Check sheet for the modelled part. Datum: model origin and axes. Units: mm. Face numbers are marked on the shaded views. A direction names the side the tool comes from. Give positions to 0.01 mm unless a question says otherwise; leave off trailing zeros. Loops run counter-clockwise (first coordinate to the right, second up) from the corner with the lowest first, then second, coordinate; pieces in that order, holes last. Notation, with made-up numbers: (-16.75, 45.25) - (1.25, 45.25) arc R8 cw to (1.25, 58.25) - close; hole circle Ø9 at (54.5, -13). An arc over 180 degrees is marked (long way). Use CSV: the item, a comma, the result in double quotes.
from build123d import *

# Parameters (mm, degrees)
SKETCH1_R           = 7
SKETCH1_R_2         = 5
SKETCH1_R_3         = 10
BOSS_EXTRUDE1_DEPTH = 5


with BuildPart() as part:
    # Sketch1 → Boss-Extrude1 (new, symmetric)
    with BuildSketch(Plane.XY):
        with BuildLine():
            ThreePointArc((27.029816197, 18.931165741), (17.392020832, 40.004906757), (15.890255583, 63.129230769))
            ThreePointArc((15.890255583, 63.129230769), (0, 81), (-15.890255583, 63.129230769))
            ThreePointArc((-15.890255583, 63.129230769), (-17.392020832, 40.004906757), (-27.029816197, 18.931165741))
            ThreePointArc((-27.029816197, 18.931165741), (-31.135684701, 10.934767406), (-32.931378534, 2.127042038))
            ThreePointArc((-32.931378534, 2.127042038), (-37.838433301, -9.754136505), (-48.963263256, -16.194613858))
            ThreePointArc((-48.963263256, -16.194613858), (-54.534765397, -32.574747935), (-37.550915036, -29.273345896))
            ThreePointArc((-37.550915036, -29.273345896), (-30.697148757, -22.889346352), (-21.566520754, -24.9776937))
            ThreePointArc((-21.566520754, -24.9776937), (-19.978209416, -26.265398313), (-18.313197236, -27.452264151))
            ThreePointArc((-18.313197236, -27.452264151), (-10.929939867, -36.447383635), (-9.804034884, -48.03))
            ThreePointArc((-9.804034884, -48.03), (0, -60), (9.804034884, -48.03))
            ThreePointArc((9.804034884, -48.03), (10.929939867, -36.447383635), (18.313197236, -27.452264151))
            ThreePointArc((18.313197236, -27.452264151), (19.978209416, -26.265398313), (21.566520754, -24.9776937))
            ThreePointArc((21.566520754, -24.9776937), (30.697148757, -22.889346352), (37.550915036, -29.273345896))
            ThreePointArc((37.550915036, -29.273345896), (54.534765397, -32.574747935), (48.963263256, -16.194613858))
            ThreePointArc((48.963263256, -16.194613858), (37.838433301, -9.754136505), (32.931378534, 2.127042038))
            ThreePointArc((32.931378534, 2.127042038), (31.135684701, 10.934767406), (27.029816197, 18.931165741))
        make_face()
        with Locations((-47, -26)):
            Circle(SKETCH1_R, mode=Mode.SUBTRACT)
        with BuildLine():
            ThreePointArc((-4.412636863, 19.507143202), (0, 20), (4.412636863, 19.507143202))
            ThreePointArc((4.412636863, 19.507143202), (7, 12.124355653), (14.687363137, 13.575027222))
            ThreePointArc((14.687363137, 13.575027222), (17.320508076, 10), (19.1, 5.93211598))
            ThreePointArc((19.1, 5.93211598), (14, 0), (19.1, -5.93211598))
            ThreePointArc((19.1, -5.93211598), (17.320508076, -10), (14.687363137, -13.575027222))
            ThreePointArc((14.687363137, -13.575027222), (7, -12.124355653), (4.412636863, -19.507143202))
            ThreePointArc((4.412636863, -19.507143202), (0, -20), (-4.412636863, -19.507143202))
            ThreePointArc((-4.412636863, -19.507143202), (-7, -12.124355653), (-14.687363137, -13.575027222))
            ThreePointArc((-14.687363137, -13.575027222), (-17.320508076, -10), (-19.1, -5.93211598))
            ThreePointArc((-19.1, -5.93211598), (-14, 0), (-19.1, 5.93211598))
            ThreePointArc((-19.1, 5.93211598), (-17.320508076, 10), (-14.687363137, 13.575027222))
            ThreePointArc((-14.687363137, 13.575027222), (-7, 12.124355653), (-4.412636863, 19.507143202))
        make_face(mode=Mode.SUBTRACT)
        with Locations((0, -50)):
            Circle(SKETCH1_R_2, mode=Mode.SUBTRACT)
        with Locations((47, -26)):
            Circle(SKETCH1_R, mode=Mode.SUBTRACT)
        with Locations((0, 65)):
            Circle(SKETCH1_R_3, mode=Mode.SUBTRACT)
    extrude(amount=BOSS_EXTRUDE1_DEPTH, both=True)


solid = part.part
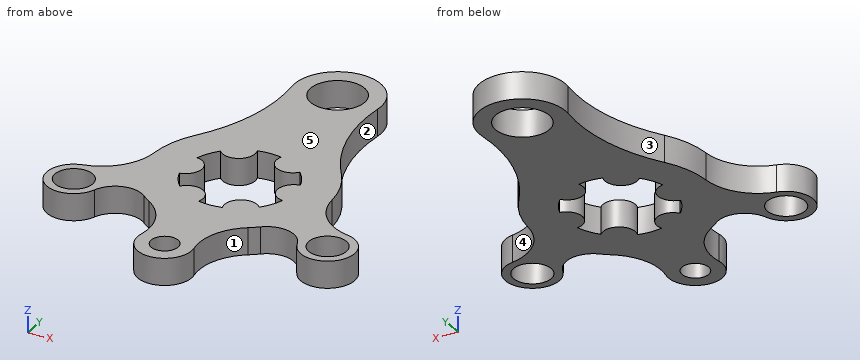
1. Go/stop test with flat-tipped pins: pin 1 Ø8 at (x, y) = (0, -50) entering from +Z; pin 2 Ø5 at (y, z) = (-19.5, 3) entering from -X; pin 3 Ø6 at (y, z) = (8, 0) entering from +X. Record where each tip stops, or that it passes through.
Completed:
pin 1,"passes through"
pin 2,"stops at x = -56.17"
pin 3,"stops at x = 32.62"
2. Sectioned sample at A-A, the plane y = -50. Record the boundary of the cut face in (x, z), and give its area (3 significant figures).
Completed:
outline,"(-10, -5) - (-5, -5) - (-5, 5) - (-10, 5) - close; (5, -5) - (10, -5) - (10, 5) - (5, 5) - close"
area,"100 mm²"
3. Release check for a two-part mould opening along Y. For the marked faces 3, 4 and 5 record: released by +Y, released by -Y, zero draft, split by the parting line, or undercut.
Completed:
face 3,"undercut"
face 4,"released by +Y"
face 5,"zero draft"
4. Sectioned sample at C-C, the plane z = -0.25. State how many separate pieces and enclosed holes the cut face has, and give its area (3 significant figures).
Completed:
separate pieces,"1"
enclosed holes,"5"
area,"4,910 mm²"
5. Sectioned sample at D-D, the plane y = 31.5. Record the boundary of the cut face in (x, z).
Completed:
outline,"(-20.18, -5) - (20.18, -5) - (20.18, 5) - (-20.18, 5) - close"
6. Set-up check for the marked faces 1 and 2: record each of +Z, -Z, +X, -X, +Y, -Y from which the full face is reachable in a straight line by a thin tool's end or side.
Completed:
face 1,"+Z, -Z"
face 2,"+Z, -Z, +X"
7. Sectioned sample at B-B, the plane x = 47. Record the boundary of the cut face in (y, z), and give its area (3 significant figures).
Completed:
outline,"(-36, -5) - (-33, -5) - (-33, 5) - (-36, 5) - close; (-19, -5) - (-15.7, -5) - (-15.7, 5) - (-19, 5) - close"
area,"63.0 mm²"
8. Scan lines: line 1 along Y through (x, z) = (0, 1.5); line 2 along Y through (x, z) = (4.5, 1.5); line 3 along X through (y, z) = (-2, 4). Record each from-to range of solid material in increasing order.
Completed:
line 1,"y = -60 to -55, -45 to -20, 20 to 55, 75 to 81"
line 2,"y = -58.93 to -52.18, -47.82 to -14.92, 14.92 to 56.07, 73.93 to 80.35"
line 3,"x = -33.64 to -14.34, 14.34 to 33.64"
